Autodesk Inventor part; units mm, degrees
ref_plane "YZ Plane" through (0, 0, 0) normal (1, 0, 0) x (0, 1, 0)
ref_plane "XZ Plane" through (0, 0, 0) normal (0, 1, 0) x (-1, 0, 0)
ref_plane "XY Plane" through (0, 0, 0) normal (0, 0, 1) x (1, 0, 0)
sketch "Sketch1" plane through (0, 0, 0) normal (0, 0, 1) x (1, 0, 0)
  line L0 (-24, 27.5) -> (24, 27.5)
  line L1 (24, 27.5) -> (24, -27.5)
  line L2 (24, -27.5) -> (-24, -27.5)
  line L3 (-24, -27.5) -> (-24, 27.5)
  line L4 (-24, 27.5) -> (24, -27.5) construction
  line L5 (24, 27.5) -> (-24, -27.5) construction
  circle A0 centre (0, 0) radius 11.5
  line L6 (-15.5, 15.5) -> (15.5, -15.5) construction
  line L7 (15.5, 15.5) -> (-15.5, -15.5) construction
  circle A1 centre (-15.5, 15.5) radius 2
  circle A2 centre (15.5, 15.5) radius 2
  circle A3 centre (-15.5, -15.5) radius 2
  circle A4 centre (15.5, -15.5) radius 2
  dimension "d0" = 48
  dimension "d1" = 55
  dimension "d2" = 23
  dimension "d3" = 31
  dimension "d4" = 31
  dimension "d5" = 4
  dimension "d6" = 4
  dimension "d7" = 4
  dimension "d8" = 4
extrude "Extrusion1" add sketch "Sketch1" along normal blind 6
sketch "Sketch2" plane through (0, 0, 6) normal (0, 0, 1) x (1, 0, 0)
  circle A0 centre (-15.5, 15.5) radius 2
  circle A1 centre (15.5, 15.5) radius 2
  circle A2 centre (15.5, -15.5) radius 2
  circle A3 centre (-15.5, -15.5) radius 2
  point P0 (0, 0)
hole "Hole1" at (-15.5, 15.5, 6) at (15.5, 15.5, 6) at (15.5, -15.5, 6) at (-15.5, -15.5, 6) direction (0, 0, -1) diameter 4 end through all counterbore diameter 10 counterbore depth 3
sketch "Sketch4" plane through (-24, 27.5, 0) normal (0, 1, 0) x (1, 0, 0)
  line L0 (0, 0) -> (0, -6)
  line L1 (0, -6) -> (48, -6)
  line L2 (48, -6) -> (48, 54)
  line L3 (48, 54) -> (0, 54)
  line L4 (0, 54) -> (0, -6)
  point P0 (24, 0)
  dimension "d20" = 60
extrude "Extrusion2" add sketch "Sketch4" along normal blind 6
sketch "Sketch5" plane through (-24, 27.5, 0) normal (0, -1, 0) x (1, 0, 0)
  arc A0 (7.75, -44) -> (12.25, -44) centre (10, -44) ccw
  line L0 (0, -54) -> (0, 0)
  line L1 (0, -27) -> (48, -27)
  line L2 (48, 6) -> (48, -54)
  line L3 (24, 0) -> (24, -54)
  line L4 (48, -54) -> (0, -54)
  arc A1 (12.25, -10) -> (7.75, -10) centre (10, -10) ccw
  line L5 (7.75, -44) -> (7.75, -10)
  line L6 (12.25, -10) -> (12.25, -44)
  arc A2 (35.75, -44) -> (40.25, -44) centre (38, -44) ccw
  arc A3 (40.25, -10) -> (35.75, -10) centre (38, -10) ccw
  line L7 (40.25, -44) -> (40.25, -10)
  line L8 (35.75, -10) -> (35.75, -44)
  dimension "d23" = 4.5
  dimension "d25" = 10
  dimension "d26" = 10
extrude "Extrusion3" cut sketch "Sketch5" against normal through all contours L5 L1 L6 A0 | L5 A1 L6 L1 | L8 A3 L7 L1 | L1 L7 A2 L8
sketch "Sketch6" plane through (-24, -27.5, 0) normal (-1, 0, 0) x (0, 0, 1)
  line L0 (6, 0) -> (6, 61)
  line L1 (6, 0) -> (0, 0)
  line L2 (-54, 55) -> (0, 55)
  line L3 (0, 0) -> (-54, 55)
  line L4 (-54, 55) -> (-54, 61)
  line L5 (-54, 61) -> (6, 61)
  line L6 (-54, 61) -> (6, 61)
  line L7 (6, 0) -> (6, 61)
  line L8 (6, 61) -> (6, 0)
  line L9 (0, 0) -> (6, 0)
  line L10 (6, 0) -> (0, 0)
  point P0 (0, 27.5)
extrude "Extrusion4" add sketch "Sketch6" against normal blind 2
ref_plane "Work Plane1" through (0, -27.5, 6) normal (-1, 0, 0) x (0, 0, 1)
mirror "Mirror1" about plane through (0, -27.5, 6) normal (-1, 0, 0) of "Extrusion4"
properties part number "CarroXY-Motor"
Part model, mm, in its own coordinate system. A direction names the side the tool comes from. Round coordinates to 2 decimals unless told otherwise and drop trailing zeros. Order: outer loops, then holes, each group sorted by start corner. A loop starts at its lowest first (then second) coordinate and runs counter-clockwise, first axis right, second up. Notation, with made-up numbers: M 72,46.5 L 76,46.5 A19 ccw 76,81.5 Z; hole C 66,68 d10. An arc over 180 degrees is marked long. Put each result on its own line as item: value. Start each with the question number.
1. Slice it at B-B on z = -14. List the corners of the cut face in (x, y), then the cut area to 3 significant figures.
2. Two-plate mould, pull along Z, no slides. Class faces 4 (the face through (18, 16, 3)), 5 (the face through (-10, 6, 0)), 6 (the face through (-11.064, -17.807, 4.479)), 7 (the face through (-16.25, 30, -27)): +Z half, -Z half, draft (parallel to the pull), parting line (faces both ways), or undercut.
3. Tool access for faces 1 (the face through (-13, 16, 3)), 2 (the face through (22, 6, -21)), 3 (the face through (13.95, 30.46, -46.25)): list every direction of +Z, -Z, +X, -X, +Y, -Y with a clear straight run to the whole face (end or side of a thin tool).
4. Slice it at A-A on x = 0. List the corners of the cut face in (y, z), then the cut area to 3 significant figures.
5. Drill centre lines: probe 1 along X at (y, z) = (-15.5, 4); probe 2 along Y at (x, z) = (15.5, 1.7); probe 3 along Y at (x, z) = (15.5, 4.7). Where is each one in solid material? Low to high. Write a range as [from, to].
6. Slice it at C-C on y = -1.5. List the corners of the cut face in (x, z), then the cut area to 3 significant figures.
7. Drop flat-ended pins along their axis: pin 1 (6.5 mm diameter, centred on x = 15.5, y = 15.5, fed in from +Z); pin 2 (11.5 mm diameter, centred on x = 15.5, y = -15.5, fed in from +Z); pin 3 (2.5 mm diameter, centred on x = -15.5, y = -15.5, fed in from -Z) (3 decimals); pin 4 (22 mm diameter, centred on x = 7.5, y = 9.5, fed in from -Z). Give the stop position or say it passes through.
8. Slice it at D-D on y = 15.5. List the corners of the cut face in (x, z), then the cut area to 3 significant figures.
Findings:
1. outline: M -24,-13.24 L -22,-13.24 L -22,27.5 L -16.25,27.5 L -16.25,33.5 L -24,33.5 Z; M -11.75,27.5 L 11.75,27.5 L 11.75,33.5 L -11.75,33.5 Z; M 16.25,27.5 L 22,27.5 L 22,-13.24 L 24,-13.24 L 24,33.5 L 16.25,33.5 Z
1. area: 397 mm2
2. face 4: +Z half
2. face 5: -Z half
2. face 6: draft
2. face 7: undercut
3. face 1: +Z
3. face 2: -Z, -Y
3. face 3: +Y, -Y
4. outline: M -27.5,0 L -11.5,0 L -11.5,6 L -27.5,6 Z; M 11.5,0 L 27.5,0 L 27.5,-54 L 33.5,-54 L 33.5,6 L 11.5,6 Z
4. area: 552 mm2
5. probe 1: [-24, -20.5], [-10.5, 10.5], [20.5, 24]
5. probe 2: [-27.5, -17.5], [-13.5, 13.5], [17.5, 33.5]
5. probe 3: [-27.5, -20.5], [-10.5, 10.5], [20.5, 33.5]
6. outline: M -24,-25.53 L -22,-25.53 L -22,0 L -11.4,0 L -11.4,6 L -24,6 Z; M 11.4,0 L 22,0 L 22,-25.53 L 24,-25.53 L 24,6 L 11.4,6 Z
6. area: 253 mm2
7. pin 1: z = 3
7. pin 2: z = 6
7. pin 3: through
7. pin 4: z = 0
8. outline: M -24,-42.22 L -22,-42.22 L -22,0 L -17.5,0 L -17.5,3 L -20.5,3 L -20.5,6 L -24,6 Z; M -13.5,0 L 13.5,0 L 13.5,3 L 10.5,3 L 10.5,6 L -10.5,6 L -10.5,3 L -13.5,3 Z; M 17.5,0 L 22,0 L 22,-42.22 L 24,-42.22 L 24,6 L 20.5,6 L 20.5,3 L 17.5,3 Z
8. area: 373 mm2
